```python
from build123d import *

# Parameters (mm, degrees)
SKETCH2_W           = 50.8
SKETCH2_H           = 25.4
BOSS_EXTRUDE1_DEPTH = 3.175
SKETCH4_W           = 33.5
SKETCH4_H           = 60
BOSS_EXTRUDE2_DEPTH = 3.175
SKETCH6_R           = 3.175
CUT_EXTRUDE2_DEPTH  = 3.175
BOSS_EXTRUDE3_DEPTH = 1.5875
SKETCH8_R           = 5.1
SKETCH8_R_2         = 1.5
CUT_EXTRUDE3_DEPTH  = 10
FILLET3_R           = 1.5


with BuildPart() as part:
    # Sketch2 → Boss-Extrude1 (new body)
    with BuildSketch(Plane(origin=(0, 0, 0), x_dir=(0, 0, -1), z_dir=(1, 0, 0))):
        Rectangle(SKETCH2_W, SKETCH2_H)
    extrude(amount=BOSS_EXTRUDE1_DEPTH)

    # Sketch4 → Boss-Extrude2 (add)
    with BuildSketch(Plane(origin=(0, 12.7, 0), x_dir=(1, 0, 0), z_dir=(0, 1, 0))):
        with Locations((16.75, 4.6)):
            Rectangle(SKETCH4_W, SKETCH4_H)
    extrude(amount=-BOSS_EXTRUDE2_DEPTH)

    # Sketch6 → Cut-Extrude2 (cut)
    with BuildSketch(Plane.ZY):
        with Locations((-12.7, 0)):
            Circle(SKETCH6_R)
        with Locations((12.7, 0)):
            Circle(SKETCH6_R)
    extrude(amount=-CUT_EXTRUDE2_DEPTH, mode=Mode.SUBTRACT)

    # Sketch7 → Boss-Extrude3 (add, symmetric)
    with BuildSketch(Plane.XY):
        Polygon((3.175, -12.7), (25.4, 9.525), (3.175, 9.525), align=None)
    extrude(amount=BOSS_EXTRUDE3_DEPTH, both=True)

    # Sketch8 → Cut-Extrude3 (cut)
    with BuildSketch(Plane(origin=(0, 12.7, 0), x_dir=(1, 0, 0), z_dir=(0, 1, 0))):
        with Locations(Location((16.75, 17.788109286, 0), (0, 0, 270))):
            Circle(SKETCH8_R)
        with Locations(Location((16.75, 7.788109286, 0), (0, 0, 270))):
            Circle(SKETCH8_R_2)
        with Locations(Location((16.75, 27.788109286, 0), (0, 0, 270))):
            Circle(SKETCH8_R_2)
        with Locations(Location((16.75, -14.014379277, 0), (0, 0, 270))):
            Circle(SKETCH8_R)
    extrude(amount=-CUT_EXTRUDE3_DEPTH, mode=Mode.SUBTRACT)

    # Fillet3
    # the kernel refuses this fillet: 1.5 mm, written as the material it adds along each edge
    with BuildSketch(Plane(origin=(4.675, 8.025, 3.0875), x_dir=(-1, 0, 0), z_dir=(0, 1, 0))) as fillet3_piece_1_section:
        Polygon((0, 0), (FILLET3_R, 0), (FILLET3_R, -FILLET3_R), (0, -FILLET3_R), align=None)
    fillet3_piece_1 = extrude(amount=FILLET3_R, mode=Mode.PRIVATE)
    fillet3_piece_1 = fillet3_piece_1 - Plane(origin=(4.675, 8.025, 3.0875), x_dir=(0.7071067811865475, 0, 0.7071067811865475), z_dir=(0, 1, 0)) * Sphere(FILLET3_R, mode=Mode.PRIVATE)
    add(fillet3_piece_1)
    with BuildSketch(Plane(origin=(4.675, 8.025, -3.0875), x_dir=(-1, 0, 0), z_dir=(0, 1, 0))) as fillet3_piece_2_section:
        Polygon((0, 0), (FILLET3_R, 0), (FILLET3_R, FILLET3_R), (0, FILLET3_R), align=None)
    fillet3_piece_2 = extrude(amount=FILLET3_R, mode=Mode.PRIVATE)
    fillet3_piece_2 = fillet3_piece_2 - Plane(origin=(4.675, 8.025, -3.0875), x_dir=(0.7071067811865475, 0, -0.7071067811865475), z_dir=(0, 1, 0)) * Sphere(FILLET3_R, mode=Mode.PRIVATE)
    add(fillet3_piece_2)
    with BuildSketch(Plane(origin=(3.175, 9.525, 25.4), x_dir=(0, -1, 0), z_dir=(0, 0, -1)), Plane(origin=(3.175, 9.525, -3.0875), x_dir=(0, -1, 0), z_dir=(0, 0, -1))) as fillet3_piece_3:
        with BuildLine():
            CenterArc((FILLET3_R, -FILLET3_R), FILLET3_R, 90, 90)
            Line((0, -FILLET3_R), (0, 0))
            Line((0, 0), (FILLET3_R, 0))
        make_face()
    extrude(amount=22.3125)
    with BuildSketch(Plane(origin=(29.15, 9.525, -1.5875), x_dir=(0, 0, -1), z_dir=(-1, 0, 0))) as fillet3_piece_4_section:
        with BuildLine():
            CenterArc((FILLET3_R, FILLET3_R), FILLET3_R, 180, 90)
            Line((0, FILLET3_R), (0, 0))
            Line((0, 0), (FILLET3_R, 0))
        make_face()
    fillet3_piece_4 = extrude(amount=24.475, mode=Mode.PRIVATE)
    fillet3_piece_4 = split(fillet3_piece_4, bisect_by=Plane(origin=(19.967902823, 4.092902823, -1.930123153), z_dir=(-0.707106781186549, 0.707106781186546, 0)), keep=Keep.TOP, mode=Mode.PRIVATE)
    add(fillet3_piece_4)
    with BuildSketch(Plane(origin=(25.4, 9.525, -1.5875), x_dir=(-0.7071067811865489, -0.7071067811865461, 0), z_dir=(0, 0, 1))) as fillet3_piece_5:
        with BuildLine():
            CenterArc((FILLET3_R * 0.414213562373, FILLET3_R), FILLET3_R, 225, 45)
            Line((-FILLET3_R * 0.292893218813, FILLET3_R * 0.292893218813), (0, 0))
            Line((0, 0), (FILLET3_R * 0.414213562373, 0))
        make_face()
    extrude(amount=3.175)
    with BuildSketch(Plane(origin=(3.175, 8.025, -1.5875), x_dir=(0, 0, -1), z_dir=(0, -1, 0))) as fillet3_piece_6_section:
        with BuildLine():
            CenterArc((FILLET3_R, FILLET3_R), FILLET3_R, 180, 90)
            Line((0, FILLET3_R), (0, 0))
            Line((0, 0), (FILLET3_R, 0))
        make_face()
    fillet3_piece_6 = extrude(amount=20.725, mode=Mode.PRIVATE)
    fillet3_piece_6 = split(fillet3_piece_6, bisect_by=Plane(origin=(8.60741784, -7.26758216, -1.930100054), z_dir=(-0.707106781186549, 0.707106781186546, 0)), keep=Keep.TOP, mode=Mode.PRIVATE)
    add(fillet3_piece_6)
    with BuildSketch(Plane(origin=(29.15, 9.525, 1.5875), x_dir=(0, 0, 1), z_dir=(-1, 0, 0))) as fillet3_piece_7_section:
        with BuildLine():
            CenterArc((FILLET3_R, -FILLET3_R), FILLET3_R, 90, 90)
            Line((0, -FILLET3_R), (0, 0))
            Line((0, 0), (FILLET3_R, 0))
        make_face()
    fillet3_piece_7 = extrude(amount=24.475, mode=Mode.PRIVATE)
    fillet3_piece_7 = split(fillet3_piece_7, bisect_by=Plane(origin=(19.967902823, 4.092902823, 1.930123153), z_dir=(-0.707106781186549, 0.707106781186546, 0)), keep=Keep.TOP, mode=Mode.PRIVATE)
    add(fillet3_piece_7)
    with BuildSketch(Plane(origin=(3.175, 8.025, 1.5875), x_dir=(0, 0, 1), z_dir=(0, -1, 0))) as fillet3_piece_8_section:
        with BuildLine():
            CenterArc((FILLET3_R, -FILLET3_R), FILLET3_R, 90, 90)
            Line((0, -FILLET3_R), (0, 0))
            Line((0, 0), (FILLET3_R, 0))
        make_face()
    fillet3_piece_8 = extrude(amount=20.725, mode=Mode.PRIVATE)
    fillet3_piece_8 = split(fillet3_piece_8, bisect_by=Plane(origin=(8.60741784, -7.26758216, 1.930100054), z_dir=(-0.707106781186549, 0.707106781186546, 0)), keep=Keep.TOP, mode=Mode.PRIVATE)
    add(fillet3_piece_8)
    with BuildSketch(Plane(origin=(25.4, 9.525, -3.140800859), x_dir=(-0.7071067811865446, -0.7071067811865503, 0), z_dir=(0, 0, 1))) as fillet3_piece_9a_section:
        with BuildLine():
            CenterArc((FILLET3_R * 0.414213562373, FILLET3_R), FILLET3_R, 225, 45)
            Line((-FILLET3_R * 0.292893218813, FILLET3_R * 0.292893218813), (0, 0))
            Line((0, 0), (FILLET3_R * 0.414213562373, 0))
        make_face()
    fillet3_piece_9a = extrude(amount=4.728300859, mode=Mode.PRIVATE)
    fillet3_piece_9a = split(fillet3_piece_9a, bisect_by=Plane(origin=(25.438403899, 9.432284787, -1.5875), z_dir=(0, 0, -1)), keep=Keep.TOP, mode=Mode.PRIVATE)
    with BuildSketch(Plane(origin=(29.15, 9.525, -1.5875), x_dir=(0, 0, -1), z_dir=(-1, 0, 0))) as fillet3_piece_9b_section:
        with BuildLine():
            CenterArc((FILLET3_R, FILLET3_R), FILLET3_R, 180, 90)
            Line((0, FILLET3_R), (0, 0))
            Line((0, 0), (FILLET3_R, 0))
        make_face()
    fillet3_piece_9b = extrude(amount=24.475, mode=Mode.PRIVATE)
    fillet3_piece_9b = split(fillet3_piece_9b, bisect_by=Plane(origin=(26.063627713, 10.188627713, -1.91198662), z_dir=(0.707106781186549, -0.707106781186546, 0)), keep=Keep.TOP, mode=Mode.PRIVATE)
    fillet3_piece_9 = fillet3_piece_9a & fillet3_piece_9b
    add(fillet3_piece_9)
    with BuildSketch(Plane(origin=(25.4, 9.525, -1.5875), x_dir=(-0.7071067811865489, -0.7071067811865461, 0), z_dir=(0, 0, 1))) as fillet3_piece_10a_section:
        with BuildLine():
            CenterArc((FILLET3_R * 0.414213562373, FILLET3_R), FILLET3_R, 225, 45)
            Line((-FILLET3_R * 0.292893218813, FILLET3_R * 0.292893218813), (0, 0))
            Line((0, 0), (FILLET3_R * 0.414213562373, 0))
        make_face()
    fillet3_piece_10a = extrude(amount=4.728300859, mode=Mode.PRIVATE)
    fillet3_piece_10a = split(fillet3_piece_10a, bisect_by=Plane(origin=(25.438403899, 9.432284787, 1.5875), z_dir=(0, 0, 1)), keep=Keep.TOP, mode=Mode.PRIVATE)
    with BuildSketch(Plane(origin=(29.15, 9.525, 1.5875), x_dir=(0, 0, 1), z_dir=(-1, 0, 0))) as fillet3_piece_10b_section:
        with BuildLine():
            CenterArc((FILLET3_R, -FILLET3_R), FILLET3_R, 90, 90)
            Line((0, -FILLET3_R), (0, 0))
            Line((0, 0), (FILLET3_R, 0))
        make_face()
    fillet3_piece_10b = extrude(amount=24.475, mode=Mode.PRIVATE)
    fillet3_piece_10b = split(fillet3_piece_10b, bisect_by=Plane(origin=(26.063627713, 10.188627713, 1.91198662), z_dir=(0.707106781186549, -0.707106781186546, 0)), keep=Keep.TOP, mode=Mode.PRIVATE)
    fillet3_piece_10 = fillet3_piece_10a & fillet3_piece_10b
    add(fillet3_piece_10)
    # the kernel refuses this fillet: 1.5 mm, written as the material it takes off along each edge
    with BuildSketch(Plane(origin=(33.5, 16.45, 25.4), x_dir=(0, 0, -1), z_dir=(0, -1, 0)), Plane(origin=(0, 16.45, -34.6), x_dir=(0, 0, 1), z_dir=(0, -1, 0)), Plane(origin=(33.5, 16.45, -34.6), x_dir=(-1, 0, 0), z_dir=(0, -1, 0)), Plane(origin=(-3.75, -12.7, -25.4), x_dir=(0, 0, 1), z_dir=(1, 0, 0))) as fillet3_2_piece_1:
        with BuildLine():
            CenterArc((FILLET3_R, -FILLET3_R), FILLET3_R, 90, 90)
            Line((0, -FILLET3_R), (0, 0))
            Line((0, 0), (FILLET3_R, 0))
        make_face()
    extrude(amount=10.675, mode=Mode.SUBTRACT)
    with BuildSketch(Plane(origin=(0, 16.45, 25.4), x_dir=(0, 0, -1), z_dir=(0, -1, 0))) as fillet3_2_piece_2:
        with BuildLine():
            CenterArc((FILLET3_R, FILLET3_R), FILLET3_R, 180, 90)
            Line((0, FILLET3_R), (0, 0))
            Line((0, 0), (FILLET3_R, 0))
        make_face()
    extrude(amount=32.9, mode=Mode.SUBTRACT)
    with BuildSketch(Plane(origin=(-3.75, -12.7, 25.4), x_dir=(0, 0, -1), z_dir=(1, 0, 0))) as fillet3_2_piece_3:
        with BuildLine():
            CenterArc((FILLET3_R, FILLET3_R), FILLET3_R, 180, 90)
            Line((0, FILLET3_R), (0, 0))
            Line((0, 0), (FILLET3_R, 0))
        make_face()
    extrude(amount=10.675, mode=Mode.SUBTRACT)


solid = part.part
```
For this review, take the finished solid that the model builds, in its own axes (mm). A direction names the side the tool comes from. Round coordinates to 2 decimals unless told otherwise and drop trailing zeros. Write each loop counter-clockwise with the first axis right and the second up, starting at its lowest first coordinate (ties: lowest second). Pieces come first, ordered by that corner, then holes.
1) Take a section at C-C on y = 11.25. Give the boundary of the cut face in (x, z).
Answer below:
outline: (0, -33.1) arc R1.5 ccw to (1.5, -34.6) - (32, -34.6) arc R1.5 ccw to (33.5, -33.1) - (33.5, 23.9) arc R1.5 ccw to (32, 25.4) - (1.5, 25.4) arc R1.5 ccw to (0, 23.9) - close; hole circle Ø10.2 at (16.75, -17.79); hole circle Ø10.2 at (16.75, 14.01); hole circle Ø3 at (16.75, -27.79); hole circle Ø3 at (16.75, -7.79)
2) Take a section at A-A on y = 0. Give the boundary of the cut face in (x, z) (1 decimal).
Answer below:
outline: (0, -25.4) - (3.2, -25.4) - (3.2, -15.9) - (0, -15.9) - close; (0, -9.5) - (3.2, -9.5) - (3.2, -3.1) arc R1.5 cw to (4.7, -1.6) - (15.9, -1.6) - (15.9, 1.6) - (4.7, 1.6) arc R1.5 cw to (3.2, 3.1) - (3.2, 9.5) - (0, 9.5) - close; (0, 15.9) - (3.2, 15.9) - (3.2, 25.4) - (1.5, 25.4) arc R1.5 ccw to (0, 23.9) - close
3) Take a section at D-D on x = 20.5. Give the boundary of the cut face in (y, z) (1 decimal), then the cut area to 3 significant figures.
Answer below:
outline: (4.6, -1.6) - (8, -1.6) arc R1.5 cw to (9.5, -3.1) - (9.5, -14.3) - (12.7, -14.3) - (12.7, 10.6) - (9.5, 10.6) - (9.5, 3.1) arc R1.5 cw to (8, 1.6) - (4.6, 1.6) - close; (9.5, -34.6) - (12.7, -34.6) - (12.7, -21.2) - (9.5, -21.2) - close; (9.5, 17.5) - (12.7, 17.5) - (12.7, 25.4) - (9.5, 25.4) - close
area: 163 mm2
4) Mouldability with a two-part tool opening along X and no side actions: class faces 1 (the face through (1.92, -12.25, 24.97)), 2 (the face through (33.05, 11.13, -34.17)), 3 (the face through (17.764, 11.135, -28.894)) as +X half, -X half, draft (parallel to the pull), parting line (faces both ways), or undercut.
Answer below:
face 1: draft
face 2: +X half
face 3: undercut
5) Take a section at B-B on z = 6. Give the boundary of the cut face in (x, y) (3 decimals).
Answer below:
outline: (0, -12.7) - (3.175, -12.7) - (3.175, 8.025) arc R1.5 cw to (4.675, 9.525) - (33.5, 9.525) - (33.5, 12.7) - (0, 12.7) - close
6) Machinability: for faces 4 (the face through (12, 10, 25.4)), 5 (the face through (0.45, 0.18, 24.97)), 6 (the face through (2, -1, -25.4)), 7 (the face through (3.6, 9.07, -14.09)), 8 (the face through (3.6, 9.07, 14.4)), which of the approach directions +Z, -Z, +X, -X, +Y, -Y give a long, thin tool a straight path to every point of the face, cutting with its end or side? Answer none if there is none.
Answer below:
face 4: +Z, +X, -X, +Y, -Y
face 5: +Z, -X, +Y, -Y
face 6: -Z, +X, -X, -Y
face 7: -Z, +X, -Y
face 8: +Z, +X, -Y
7) For line 1 along Y through (x, z) = (2.2, 12.7) (3 decimals); line 2 along X through (y, z) = (-3.75, -4.5) (3 decimals); line 3 along Y through (x, z) = (18, -23) (3 decimals), list the stretches that pass through material, from the lowest coordinate up.
Answer below:
line 1: y = -12.7 to -3.175, 3.175 to 12.7
line 2: x = 0 to 3.175
line 3: y = 9.525 to 12.7
8) Insertion check: pin 1 Ø6 at (y, z) = (1.5, -11.5) entering from +X (3 decimals); pin 2 Ø5 at (x, z) = (16.75, -7.79) entering from -Y (3 decimals); pin 3 Ø2 at (x, z) = (15, -19.5) entering from -Y; pin 4 Ø9.5 at (x, y) = (10.5, -3) entering from +Z. Each pin has a flat end and moves straight along its axis. Give the tip position at first contact, or say it passes through.
Answer below:
pin 1: stops at x = 3.175
pin 2: stops at y = 9.525
pin 3: passes through
pin 4: stops at z = 1.59
